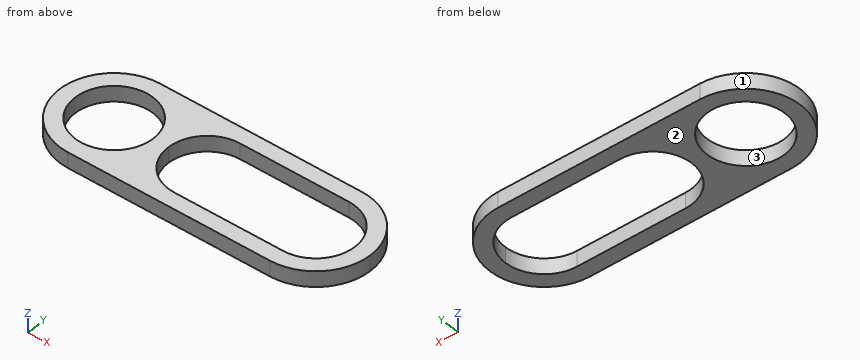
from build123d import *

# Parameters (mm, degrees)
F0_R     = 2.5
F2_DEPTH = 1


with BuildPart() as f2:
    # F0 (on Top) → F2 (new body)
    with BuildSketch(Plane.XY):
        with BuildLine():
            ThreePointArc((6, -2.5), (4.232233047, -1.767766953), (3.5, 0))
            ThreePointArc((3.5, 0), (2.4748737342, -2.4748737342), (0, -3.5))
            Line((0, -3.5), (13, -3.5))
            ThreePointArc((13, -3.5), (11.6771243445, -3.2403703492), (10.5505102572, -2.5))
            Line((10.5505102572, -2.5), (6, -2.5))
        make_face()
        with BuildLine():
            ThreePointArc((16.5, 0), (15.4748737342, 2.4748737342), (13, 3.5))
            ThreePointArc((13, 3.5), (11.6771243445, 3.2403703492), (10.5505102572, 2.5))
            Line((10.5505102572, 2.5), (13, 2.5))
            ThreePointArc((13, 2.5), (14.767766953, 1.767766953), (15.5, 0))
            ThreePointArc((15.5, 0), (14.767766953, -1.767766953), (13, -2.5))
            Line((13, -2.5), (10.5505102572, -2.5))
            ThreePointArc((10.5505102572, -2.5), (11.6771243445, -3.2403703492), (13, -3.5))
            ThreePointArc((13, -3.5), (15.4748737342, -2.4748737342), (16.5, 0))
        make_face()
        with BuildLine():
            ThreePointArc((0, 3.5), (2.4748737342, 2.4748737342), (3.5, 0))
            ThreePointArc((3.5, 0), (4.232233047, 1.767766953), (6, 2.5))
            Line((6, 2.5), (10.5505102572, 2.5))
            ThreePointArc((10.5505102572, 2.5), (11.6771243445, 3.2403703492), (13, 3.5))
            Line((13, 3.5), (0, 3.5))
        make_face()
        with BuildLine():
            ThreePointArc((0, -3.5), (2.4748737342, -2.4748737342), (3.5, 0))
            ThreePointArc((3.5, 0), (2.4748737342, 2.4748737342), (0, 3.5))
            ThreePointArc((0, 3.5), (-3.5, 0), (0, -3.5))
        make_face()
        Circle(F0_R, mode=Mode.SUBTRACT)
    extrude(amount=F2_DEPTH)


solid = f2.part
Can you work these out from the model? Positions are in its coordinate system, mm. Face numbers are marked on the shaded views. Give positions to 0.01 mm unless a question says otherwise; leave off trailing zeros. Loops run counter-clockwise (first coordinate to the right, second up) from the corner with the lowest first, then second, coordinate; pieces in that order, holes last. Notation, with made-up numbers: (-28, -30) - (30, -30) arc R22 cw to (30, -16) - close; hole circle Ø6 at (56.5, 40). An arc over 180 degrees is marked (long way). Return JSON: item names as keys, results as strings.
1. I want a section at C-C on y = -2. Please give me the cut outline in (x, z).
Output values:
{"outline": "(-2.87, 0) - (-1.5, 0) - (-1.5, 1) - (-2.87, 1) - close; (1.5, 0) - (4.5, 0) - (4.5, 1) - (1.5, 1) - close; (14.5, 0) - (15.87, 0) - (15.87, 1) - (14.5, 1) - close"}
2. I want a section at D-D on y = -1. Please give me the cut outline in (x, z), and give its area (3 significant figures).
Output values:
{"outline": "(-3.35, 0) - (-2.29, 0) - (-2.29, 1) - (-3.35, 1) - close; (2.29, 0) - (3.71, 0) - (3.71, 1) - (2.29, 1) - close; (15.29, 0) - (16.35, 0) - (16.35, 1) - (15.29, 1) - close", "area": "3.54 mm²"}
3. We'd pull the mould along Y, two halves only. Please class the marked faces 1, 2 and 3: +Y half, -Y half, draft (parallel to the pull), parting line (faces both ways), or undercut.
Output values:
{"face 1": "parting line", "face 2": "draft", "face 3": "undercut"}
4. I want a section at B-B on x = 8.5. Please give me the cut outline in (y, z).
Output values:
{"outline": "(-3.5, 0) - (-2.5, 0) - (-2.5, 1) - (-3.5, 1) - close; (2.5, 0) - (3.5, 0) - (3.5, 1) - (2.5, 1) - close"}
5. If I drill on line 1 (X direction, y = 1.5, z = 0.7); line 2 (Y direction, x = 0, z = 0.6); line 3 (X direction, y = -1, z = 0.5), over which ranges is the centre line in solid material (lowest first)?
Output values:
{"line 1": "x = -3.16 to -2, 2 to 4, 15 to 16.16", "line 2": "y = -3.5 to -2.5, 2.5 to 3.5", "line 3": "x = -3.35 to -2.29, 2.29 to 3.71, 15.29 to 16.35"}
6. I want a section at A-A on z = 0.7. Please give me the cut outline in (x, y), and give its area (3 significant figures).
Output values:
{"outline": "(0, -3.5) - (13, -3.5) arc R3.5 ccw to (13, 3.5) - (0, 3.5) arc R3.5 ccw to start; hole circle Ø5 at (0, 0); hole (6, -2.5) - (13, -2.5) arc R2.5 ccw to (13, 2.5) - (6, 2.5) arc R2.5 ccw to start", "area": "55.2 mm²"}
